from build123d import *

# Parameters (mm, degrees)
SKETCH2_R           = 60
SKETCH2_R_2         = 5
BOSS_EXTRUDE1_DEPTH = 10
SKETCH3_R           = 5
CUT_EXTRUDE1_DEPTH  = 32
SKETCH4_R           = 81.078971207
CUT_EXTRUDE2_DEPTH  = 130


with BuildPart() as part:
    # Sketch2 → Boss-Extrude1 (new body)
    with BuildSketch(Plane.XY):
        Circle(SKETCH2_R)
        Circle(SKETCH2_R_2, mode=Mode.SUBTRACT)
    extrude(amount=BOSS_EXTRUDE1_DEPTH)

    # Sketch3 → Cut-Extrude1 (cut)
    with BuildSketch(Plane.XY.offset(10)):
        with Locations((45, 0)):
            Circle(SKETCH3_R)
    extrude(amount=-CUT_EXTRUDE1_DEPTH, mode=Mode.SUBTRACT)

    # Sketch4 → Cut-Extrude2 (cut)
    with BuildSketch(Plane(origin=(0, 0, 0), x_dir=(-1, 0, 0), z_dir=(0, 0, -1))):
        Circle(SKETCH4_R)
        with BuildLine():
            Line((-5.781451877, -24.322311037), (-45, -15))
            ThreePointArc((-45, -15), (-59.905960926, -1.676999964), (-48.332972793, 14.625022816))
            Line((-48.332972793, 14.625022816), (-5.781451877, 24.322311037))
            ThreePointArc((-5.781451877, 24.322311037), (25, 0), (-5.781451877, -24.322311037))
        make_face(mode=Mode.SUBTRACT)
    extrude(amount=-CUT_EXTRUDE2_DEPTH, mode=Mode.SUBTRACT)


solid = part.part
Verification items for the finished model (mm, model axes). Round coordinates to 2 decimals unless told otherwise and drop trailing zeros. Loops run counter-clockwise (first coordinate to the right, second up) from the corner with the lowest first, then second, coordinate; pieces in that order, holes last. Notation, with made-up numbers: (-27.75, -12) - (27.25, -12) arc R19 ccw to (27.25, 14) - close; hole circle Ø3 at (68, -5.75). An arc over 180 degrees is marked (long way). Answer in a Markdown table with one row per item. Add a question column.
Q1. Section check C-C on z = 6. Enter the section's corners in (x, y).
Q2. Release check for a two-part mould opening along Y. For faces 1 (the face through (17, 0, 0)), 2 (the face through (40, 0, 5)), 3 (the face through (59.87, -1.98, 4.93)) record: pulls with the +Y half, pulls with the -Y half, needs draft (parallel to the pull), parting line crosses it, or undercut.
Q3. Gauge pin test, flat ends, axial feed: pin 1 (1 mm diameter, centred on y = 10.5, z = 9, fed in from +X); pin 2 (1 mm diameter, centred on x = 14.5, z = 6.5, fed in from +Y); pin 3 (2 mm diameter, centred on x = -13, z = 9, fed in from -Y). Record the tip position at first contact, or that the pin passes through.
Q4. Section check B-B on x = 0. Enter the section's corners in (y, z), plus the area to 3 significant figures.
Q5. Section check D-D on x = 24.5. Enter the section's corners in (y, z).
Q6. Material ranges on line 1 (Y direction, x = 0, z = 4); line 2 (Y direction, x = 45, z = 6); line 3 (Y direction, x = -5.5, z = 7), recorded low to high.
Q7. Section check A-A on y = 0. Enter the section's corners in (x, z).
Found:
| question | item | result |
|---|---|---|
| 1 | outline | (5.78, -24.32) - (45, -15) arc R15 ccw to (48.33, 14.63) - (5.78, 24.32) arc R25 ccw (long way) to start; hole circle Ø10 at (0, 0); hole circle Ø10 at (45, 0) |
| 2 | face 1 | needs draft |
| 2 | face 2 | undercut |
| 2 | face 3 | parting line crosses it |
| 3 | pin 1 | stops at x = 56.18 |
| 3 | pin 2 | stops at y = 22.45 |
| 3 | pin 3 | stops at y = -21.93 |
| 4 | outline | (-25, 0) - (-5, 0) - (-5, 10) - (-25, 10) - close; (5, 0) - (25, 0) - (25, 10) - (5, 10) - close |
| 4 | area | 400 mm² |
| 5 | outline | (-19.87, 0) - (20.06, 0) - (20.06, 10) - (-19.87, 10) - close |
| 6 | line 1 | y = -25 to -5, 5 to 25 |
| 6 | line 2 | y = -15 to -5, 5 to 15.38 |
| 6 | line 3 | y = -24.39 to 24.39 |
| 7 | outline | (-25, 0) - (-5, 0) - (-5, 10) - (-25, 10) - close; (5, 0) - (40, 0) - (40, 10) - (5, 10) - close; (50, 0) - (60, 0) - (60, 10) - (50, 10) - close |
